Source: CAD feature listing. Evaluate the final solid. Frame: model axes, mm. A direction names the side the tool comes from. Give positions to 0.01 mm unless a question says otherwise; leave off trailing zeros. Loops run counter-clockwise (first coordinate to the right, second up) from the corner with the lowest first, then second, coordinate; pieces in that order, holes last. Notation, with made-up numbers: (23.5, 63.25) -> (54.5, 63.25) arc R36 cw to (54.5, 101.25) -> close; hole circle Ø11 at (-19, 26.25). An arc over 180 degrees is marked (long way). Return JSON: item names as keys, results as strings. Group by question number.
```python
from build123d import *

# Parameters (mm, degrees)
BOSS_EXTRUDE1_DEPTH  = 17.5
BOSS_EXTRUDE2_DEPTH  = 6.5
SKETCH4_W            = 24.52025143
SKETCH4_H            = 31.2
CUT_EXTRUDE1_DEPTH   = 3.5
FILLET1_R            = 5
SKETCH7_W            = 10
SKETCH7_H            = 4
BOSS_EXTRUDE3_DEPTH  = 6.5
FILLET2_R            = 1
SKETCH8_W            = 18
SKETCH8_H            = 20
CUT_EXTRUDE4_DEPTH   = 66.139506352
FILLET3_R            = 0.5
CUT_EXTRUDE7_DEPTH   = 2.5
M3_CLEARANCE_HOLE1_D = 3.6
SKETCH14_W           = 24.52025143
SKETCH14_H           = 3.75
CUT_EXTRUDE8_DEPTH   = 48.880627126


with BuildPart() as part:
    # Sketch1 → Boss-Extrude1 (new body)
    with BuildSketch(Plane.XY):
        Polygon((-27.260125715, 5.300000005), (-12.260125715, 5.300000005), (-12.260125715, 36.500000005), (12.260125715, 36.500000005), (12.260125715, 5.300000005), (27.260125715, 5.300000005), (27.260125715, 9.300000005), (17.260125715, 9.300000005), (17.260125715, 38.858678923), (17.260125715, 41.050000005), (15.150659775, 41.050000005), (12, 41.050000005), (-12, 41.050000005), (-17.260125715, 41.050000005), (-17.260125715, 39.558678923), (-17.260125715, 9.300000005), (-27.260125715, 9.300000005), align=None)
    extrude(amount=BOSS_EXTRUDE1_DEPTH)

    # Sketch2 → Boss-Extrude2 (add)
    with BuildSketch(Plane.XY.offset(17.5)):
        Polygon((-17.260125715, 9.300000005), (-17.260125715, 41.050000005), (17.260125715, 41.050000005), (17.260125715, 5.300000005), (-17.260125715, 5.300000005), align=None)
    extrude(amount=BOSS_EXTRUDE2_DEPTH)

    # Sketch4 → Cut-Extrude1 (cut)
    with BuildSketch(Plane(origin=(0, 0, 17.5), x_dir=(-1, 0, 0), z_dir=(0, 0, -1))):
        with Locations((0, 20.900000005)):
            Rectangle(SKETCH4_W, SKETCH4_H)
    extrude(amount=-CUT_EXTRUDE1_DEPTH, mode=Mode.SUBTRACT)

    # Fillet1
    fillet1_edges = [part.edges().sort_by_distance(p)[0] for p in [
        (-17.260125715, 41.050000005, 12),
        (17.260125715, 41.050000005, 12),
    ]]
    fillet(fillet1_edges, radius=FILLET1_R)

    # Sketch7 → Boss-Extrude3 (add, through all)
    with BuildSketch(Plane.XY.offset(17.5)):
        with Locations((-22.260125715, 7.300000005)):
            Rectangle(SKETCH7_W, SKETCH7_H)
        with Locations((22.260125715, 7.300000005)):
            Rectangle(SKETCH7_W, SKETCH7_H)
    extrude(amount=BOSS_EXTRUDE3_DEPTH)

    # Fillet2
    fillet2_edges = [part.edges().sort_by_distance(p)[0] for p in [
        (12.260125715, 20.900000005, 0),
        (-12.260125715, 20.900000005, 0),
    ]]
    fillet(fillet2_edges, radius=FILLET2_R)

    # Sketch8 → Cut-Extrude4 (cut, through all)
    with BuildSketch(Plane.ZY.offset(17.260125715)):
        with Locations((12, 21.300000005)):
            Rectangle(SKETCH8_W, SKETCH8_H)
    extrude(amount=-CUT_EXTRUDE4_DEPTH, mode=Mode.SUBTRACT)

    # Fillet3
    fillet3_edges = [part.edges().sort_by_distance(p)[0] for p in [
        (12.260125715, 8.300000005, 21),
        (12.260125715, 21.300000005, 3),
        (17.260125715, 21.300000005, 3),
        (-12.260125715, 21.300000005, 3),
        (17.260125715, 21.300000005, 21),
        (17.260125715, 31.300000005, 12),
        (17.260125715, 11.300000005, 12),
        (14.760125715, 11.300000005, 21),
        (12.260125715, 11.300000005, 12),
        (-12.260125715, 11.300000005, 12),
        (-14.760125715, 11.300000005, 21),
        (-17.260125715, 21.300000005, 3),
        (-17.260125715, 11.300000005, 12),
        (-17.260125715, 21.300000005, 21),
        (-17.260125715, 31.300000005, 12),
        (-12.260125715, 8.300000005, 21),
    ]]
    fillet(fillet3_edges, radius=FILLET3_R)

    # Sketch6 → Cut-Extrude7 (cut)
    with BuildSketch(Plane(origin=(0, 9.300000005, 0), x_dir=(1, 0, 0), z_dir=(0, 1, 0))):
        Polygon((22.25, -1.24722325), (25.5, -3.123611625), (25.5, -6.876388375), (22.25, -8.75277675), (19, -6.876388375), (19, -3.123611625), align=None)
        Polygon((22.25, -22.75277675), (25.5, -20.876388375), (25.5, -17.123611625), (22.25, -15.24722325), (19, -17.123611625), (19, -20.876388375), align=None)
        Polygon((-22.25, -8.75277675), (-19, -6.876388375), (-19, -3.123611625), (-22.25, -1.24722325), (-25.5, -3.123611625), (-25.5, -6.876388375), align=None)
        Polygon((-22.25, -15.24722325), (-19, -17.123611625), (-19, -20.876388375), (-22.25, -22.75277675), (-25.5, -20.876388375), (-25.5, -17.123611625), align=None)
    extrude(amount=-CUT_EXTRUDE7_DEPTH, mode=Mode.SUBTRACT)

    # M3 Clearance Hole1 (through all)
    with Locations(Plane(origin=(0, 9.300000005, 0), x_dir=(1, 0, 0), z_dir=(0, 1, 0))):
        with Locations((22.25, -19), (22.25, -5), (-22.25, -5), (-22.25, -19)):
            Hole(M3_CLEARANCE_HOLE1_D / 2)

    # Sketch14 → Cut-Extrude8 (cut, through all)
    with BuildSketch(Plane.XZ.offset(-36.500000005)):
        with Locations((0, 19.125)):
            Rectangle(SKETCH14_W, SKETCH14_H)
    extrude(amount=-CUT_EXTRUDE8_DEPTH, mode=Mode.SUBTRACT)


solid = part.part
```
1) Contact query for flat-ended pins moving along their axis: P1, Ø10, axis at y = 16.5, z = 13, coming from the +X side; P2, Ø6, axis at x = 22.25, z = 5, coming from the -Y side; P3, Ø5, axis at x = 23.5, z = 17.5, coming from the +Y side; P4, Ø1.5, axis at x = -4, z = 2.5, coming from the -Y side. Output: stop coordinate, or through.
2) Cut plane C-C on z = 11.5. Return loops of the section in (x, y), then the cut area to 3 significant figures.
3) Cut plane B-B on y = 24. Return loops of the section in (x, z), then the cut area to 3 significant figures.
4) Reachability of faces 4 (the face through (-23.9, 8.1, 16.2)), 5 (the face through (-17.26, 33, 13)), 6 (the face through (0, 41.05, 9)) from +Z, -Z, +X, -X, +Y, -Y: full face, straight path, thin tool, end or side. Return the list, or none.
5) Cut plane D-D on z = 19. Count the separate pieces of the cut face and the enclosed holes in it, then the cut area to 3 significant figures.
6) Material intervals for line 1 (X direction, y = 6.1, z = 19); line 2 (Z direction, x = -22.25, y = 6); line 3 (X direction, y = 13.5, z = 2.5), sorted ascending.
7) Mould query, pull axis Y, two halves, no side actions, for faces 1 (the face through (-15, 21, 3)), 2 (the face through (-20.6, 8.1, 7.8)), 3 (the face through (22, 9.3, 12)). Classes: released by +Y, released by -Y, zero draft, split by the parting line, or undercut.
8) Cut plane A-A on x = -1. Return loops of the section in (y, z).
Calculated:
{
 "1": {"P1": "through", "P2": "y = 5.3", "P3": "y = 9.3", "P4": "y = 36.5"},
 "2": {"outline": "(-27.26, 5.3) -> (-12.26, 5.3) -> (-12.26, 10.8) arc R0.5 ccw to (-12.76, 11.3) -> (-16.76, 11.3) arc R0.5 ccw to (-17.26, 10.8) -> (-17.26, 9.3) -> (-27.26, 9.3) -> close; (-17.26, 31.8) arc R0.5 ccw to (-16.76, 31.3) -> (-12.26, 31.3) -> (-12.26, 36.5) -> (12.26, 36.5) -> (12.26, 31.3) -> (16.76, 31.3) arc R0.5 ccw to (17.26, 31.8) -> (17.26, 36.05) arc R5 ccw to (12.26, 41.05) -> (-12.26, 41.05) arc R5 ccw to (-17.26, 36.05) -> close; (12.26, 5.3) -> (27.26, 5.3) -> (27.26, 9.3) -> (17.26, 9.3) -> (17.26, 10.8) arc R0.5 ccw to (16.76, 11.3) -> (12.76, 11.3) arc R0.5 ccw to (12.26, 10.8) -> close", "area": "338 mm2"},
 "3": {"outline": "(-17.26, 0) -> (-13.26, 0) arc R1 ccw to (-12.26, 1) -> (-12.26, 2.5) arc R0.5 ccw to (-12.76, 3) -> (-16.76, 3) arc R0.5 ccw to (-17.26, 2.5) -> close; (-17.26, 21.5) arc R0.5 ccw to (-16.76, 21) -> (16.76, 21) arc R0.5 ccw to (17.26, 21.5) -> (17.26, 24) -> (-17.26, 24) -> close; (12.26, 1) arc R1 ccw to (13.26, 0) -> (17.26, 0) -> (17.26, 2.5) arc R0.5 ccw to (16.76, 3) -> (12.76, 3) arc R0.5 ccw to (12.26, 2.5) -> close", "area": "133 mm2"},
 "4": {"face 4": "+Y", "face 5": "+Z, -Z, -X, +Y", "face 6": "+Z, -Z, +X, -X, +Y"},
 "5": {"separate pieces": "6", "enclosed holes": "0", "area": "183 mm2"},
 "6": {"line 1": "-27.26 to -24.05, -20.45 to -12.26, 12.26 to 20.45, 24.05 to 27.26", "line 2": "0 to 3.2, 6.8 to 17.2, 20.8 to 24", "line 3": "-17.26 to -12.26, 12.26 to 17.26"},
 "7": {"face 1": "undercut", "face 2": "zero draft", "face 3": "released by +Y"},
 "8": {"outline": "(5.3, 21) -> (41.05, 21) -> (41.05, 24) -> (5.3, 24) -> close; (36.5, 0) -> (41.05, 0) -> (41.05, 17.25) -> (36.5, 17.25) -> close"}
}
